Design review of the part built by this model. Coordinates are the model's own, in mm. A direction names the side the tool comes from. Coordinates: 2 decimals unless noted, no trailing zeros. Order: outer loops, then holes, each group sorted by start corner. A loop starts at its lowest first (then second) coordinate and runs counter-clockwise, first axis right, second up. Notation, with made-up numbers: M 2,-32 L 45,-32 A33 cw 45,1 Z; hole C 1.5,41.25 d2. An arc over 180 degrees is marked long. Answer in a Markdown table with one row per item.
Autodesk Inventor part; units mm, degrees
ref_plane "YZ Plane" through (0, 0, 0) normal (1, 0, 0) x (0, 1, 0)
ref_plane "XZ Plane" through (0, 0, 0) normal (0, 1, 0) x (-1, 0, 0)
ref_plane "XY Plane" through (0, 0, 0) normal (0, 0, 1) x (1, 0, 0)
sketch "Sketch1" plane through (0, 0, 0) normal (0, 1, 0) x (-1, 0, 0)
  line L0 (1.5625, 15) -> (-1.5625, 15)
  line L1 (-1.5625, 15) -> (-1.5625, -15)
  line L2 (-1.5625, -15) -> (1.5625, -15)
  line L3 (1.5625, -15) -> (1.5625, 15)
  line L4 (1.5625, 15) -> (-1.5625, -15) construction
  line L5 (-1.5625, 15) -> (1.5625, -15) construction
  point P0 (0, 0)
  dimension "d0" = 3.125
  dimension "d1" = 30
extrude "Extrusion1" add sketch "Sketch1" along normal blind 17
sketch "Sketch3" plane through (0, 17, 0) normal (0, 1, 0) x (1, 0, 0)
  line L0 (-1.5625, -9.99) -> (1.5625, -9.99)
  line L1 (1.5625, -9.99) -> (1.5625, 9.99)
  line L2 (1.5625, 9.99) -> (-1.5625, 9.99)
  line L3 (-1.5625, 9.99) -> (-1.5625, -9.99)
  line L4 (-1.5625, -9.99) -> (1.5625, 9.99) construction
  line L5 (1.5625, -9.99) -> (-1.5625, 9.99) construction
  point P0 (0, 0)
  dimension "d4" = 3.125
  dimension "d5" = 19.98
extrude "Extrusion2" add sketch "Sketch3" along normal blind 3.1
sketch "Sketch4" plane through (0, 0, 0) normal (0, -1, 0) x (1, 0, 0)
  line L0 (-1.5625, 15) -> (1.5625, 15)
  line L1 (-1.5625, -15) -> (-1.5625, -9.99)
  line L2 (1.5625, 15) -> (-1.5625, 15)
  line L3 (-1.5625, 15) -> (-1.5625, -15)
  line L4 (-1.5625, -15) -> (1.5625, -15)
  line L5 (1.5625, -15) -> (1.5625, 15)
  point P0 (0, 0)
extrude "Extrusion3" add sketch "Sketch4" along normal blind 11
properties part number "bate2_3DPrint"
(1) Add section A-A, the plane x = 0.9. Give the boundary of the cut face in (y, z), and give its area (3 significant figures).
Return value:
| item | result |
|---|---|
| outline | M -11,-15 L 17,-15 L 17,-9.99 L 20.1,-9.99 L 20.1,9.99 L 17,9.99 L 17,15 L -11,15 Z |
| area | 902 mm2 |
(2) For line 1 along Z through (x, y) = (0.7, 18); line 2 along Y through (x, z) = (0.85, 13.25), list the stretches that pass through material, from the lowest coordinate up. Write a range as from..to.
Return value:
| item | result |
|---|---|
| line 1 | z = -9.99..9.99 |
| line 2 | y = -11..17 |
(3) For faces 1 (the flat face through (0, 20.1, 0)), 2 (the flat face through (0, 19, 9.99)), 3 (the flat face through (0, 17, -12)), list the 3-axis set-ups (+Z, -Z, +X, -X, +Y, -Y) from which the entire face can be reached by the end or side of a thin tool; tool diameter is ignored.
Return value:
| item | result |
|---|---|
| face 1 | +Z, -Z, +X, -X, +Y |
| face 2 | +Z, +X, -X, +Y |
| face 3 | -Z, +X, -X, +Y |
(4) Add section B-B, the plane y = 18. Give the boundary of the cut face in (x, z), and give its area (3 significant figures).
Return value:
| item | result |
|---|---|
| outline | M -1.56,-9.99 L 1.56,-9.99 L 1.56,9.99 L -1.56,9.99 Z |
| area | 62.4 mm2 |
(5) Add section C-C, the plane z = 13.25. Give the boundary of the cut face in (x, y), and give its area (3 significant figures).
Return value:
| item | result |
|---|---|
| outline | M -1.56,-11 L 1.56,-11 L 1.56,17 L -1.56,17 Z |
| area | 87.5 mm2 |
(6) Insertion check: pin 1 Ø0.9 at (x, y) = (-0.5, 19) entering from +Z; pin 2 Ø1.6 at (x, z) = (-0.5, -13.5) entering from +Y. Each pin has a flat end and moves straight along its axis. Give the tip position at first contact, or say it passes through.
Return value:
| item | result |
|---|---|
| pin 1 | stops at z = 9.99 |
| pin 2 | stops at y = 17 |
